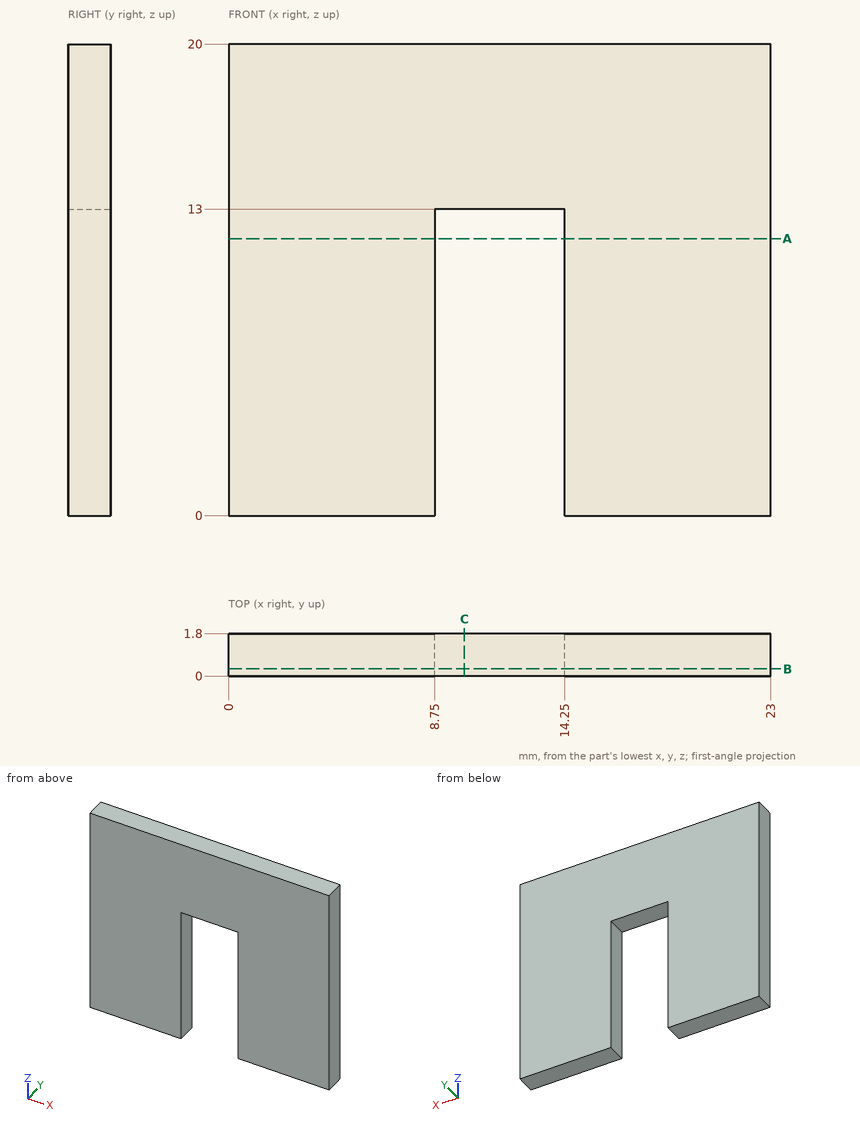
Input: dimensioned drawing with shaded views. Units: mm. Origin: part minimum x, y, z. Round coordinates to 2 decimals unless told otherwise and drop trailing zeros. Loops run counter-clockwise (first coordinate to the right, second up) from the corner with the lowest first, then second, coordinate; pieces in that order, holes last. Notation, with made-up numbers: (-24, 87) -> (20, 87) arc R11 cw to (20, 99) -> close; hole circle Ø1 at (-30, -36). An arc over 180 degrees is marked (long way). Answer as a JSON object with one key per item and string values. Group by question number.
Q1. Section query B-B (y = 0.3). Output: boundary loops of the cut face in (x, z), plus the area to 4 significant figures.
Q2. Ray query, line 1 (X direction, y = 0.7, z = 6); line 2 (Z direction, x = 14, y = 1.5). Return the intervals inside material, ascending. Write a range as from..to.
Q3. Section query A-A (z = 11.75). Output: boundary loops of the cut face in (x, y), plus the area to 3 significant figures.
Q4. Section query C-C (x = 10). Output: boundary loops of the cut face in (y, z), plus the area to 3 significant figures.
Q5. Contact query for a flat-ended pin moving along its axis: P1, Ø0.9, axis at x = 12, y = 1.5, coming from the -Z side. Output: stop coordinate, or through.
Completed:
{
 "1": {"outline": "(0, 0) -> (8.75, 0) -> (8.75, 13) -> (14.25, 13) -> (14.25, 0) -> (23, 0) -> (23, 20) -> (0, 20) -> close", "area": "388.5 mm²"},
 "2": {"line 1": "0..8.75, 14.25..23", "line 2": "13..20"},
 "3": {"outline": "(0, 0) -> (8.75, 0) -> (8.75, 1.8) -> (0, 1.8) -> close; (14.25, 0) -> (23, 0) -> (23, 1.8) -> (14.25, 1.8) -> close", "area": "31.5 mm²"},
 "4": {"outline": "(0, 13) -> (1.8, 13) -> (1.8, 20) -> (0, 20) -> close", "area": "12.6 mm²"},
 "5": {"P1": "z = 13"}
}
